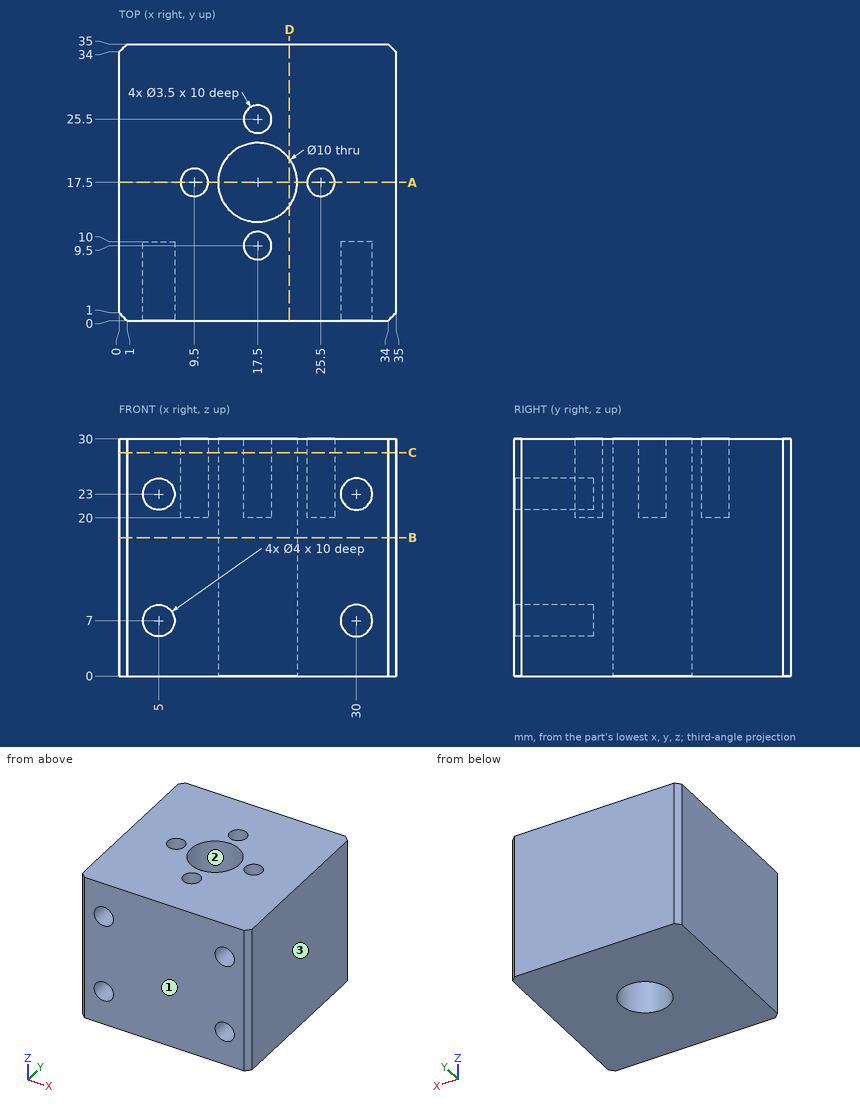
Design review of the part shown in the three views and the two pictorial views. Dimensions are in mm from the part's minimum x, y and z. Coordinates: 2 decimals unless noted, no trailing zeros. Loops run counter-clockwise (first coordinate to the right, second up) from the corner with the lowest first, then second, coordinate; pieces in that order, holes last.
(1) Consider section C-C, the plane z = 28.25. Give the boundary of the cut face in (x, y).
Determined:
outline: (0, 1) - (1, 0) - (34, 0) - (35, 1) - (35, 34) - (34, 35) - (1, 35) - (0, 34) - close; hole circle Ø3.5 at (9.5, 17.5); hole circle Ø10 at (17.5, 17.5); hole circle Ø3.5 at (17.5, 9.5); hole circle Ø3.5 at (17.5, 25.5); hole circle Ø3.5 at (25.5, 17.5)
(2) Draft analysis for pull direction Y (two halves, no side actions). For the marked faces 1, 2 and 3, state which applies: +Y half, -Y half, draft (parallel to the pull), parting line (faces both ways), or undercut.
Determined:
face 1: -Y half
face 2: undercut
face 3: draft
(3) Insertion check: P1, Ø3.5, axis at x = 30, z = 7, coming from the -Y side; P2, Ø1.8, axis at x = 10, y = 17, coming from the +Z side. Each pin has a flat end and moves straight along its axis. Give the tip position at first contact, or say it passes through.
Determined:
P1: stops at y = 10
P2: stops at z = 20
(4) Consider section D-D, the plane x = 21.5. Give the boundary of the cut face in (y, z), plus the area to 3 significant figures.
Determined:
outline: (0, 0) - (14.5, 0) - (14.5, 30) - (0, 30) - close; (20.5, 0) - (35, 0) - (35, 30) - (20.5, 30) - close
area: 870 mm2
(5) Consider section B-B, the plane z = 17.5. Give the boundary of the cut face in (x, y), plus the area to 3 significant figures.
Determined:
outline: (0, 1) - (1, 0) - (34, 0) - (35, 1) - (35, 34) - (34, 35) - (1, 35) - (0, 34) - close; hole circle Ø10 at (17.5, 17.5)
area: 1,140 mm2
(6) Consider section A-A, the plane y = 17.5. Give the boundary of the cut face in (x, z).
Determined:
outline: (0, 0) - (12.5, 0) - (12.5, 30) - (11.25, 30) - (11.25, 20) - (7.75, 20) - (7.75, 30) - (0, 30) - close; (22.5, 0) - (35, 0) - (35, 30) - (27.25, 30) - (27.25, 20) - (23.75, 20) - (23.75, 30) - (22.5, 30) - close
(7) Wall thickness on L1, parallel to Z at x = 30, y = 7.25; L2, parallel to Y at x = 17.5, z = 24.5; L3, parallel to Y at x = 9.5, z = 25: over which ranges is each line inside the solid? List them lowest first.
Determined:
L1: z = 0 to 5, 9 to 21, 25 to 30
L2: y = 0 to 7.75, 11.25 to 12.5, 22.5 to 23.75, 27.25 to 35
L3: y = 0 to 15.75, 19.25 to 35
